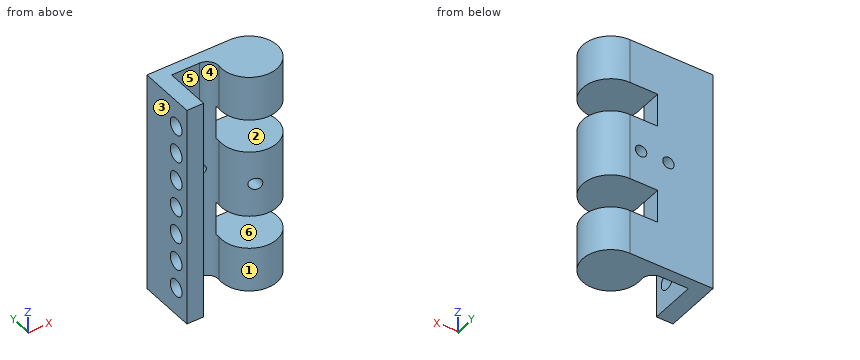
Autodesk Inventor part; units mm, degrees
ref_plane "YZ Plane" through (0, 0, 0) normal (1, 0, 0) x (0, 1, 0)
ref_plane "XZ Plane" through (0, 0, 0) normal (0, 1, 0) x (-1, 0, 0)
ref_plane "XY Plane" through (0, 0, 0) normal (0, 0, 1) x (1, 0, 0)
sketch "Sketch1" plane through (0, 0, 0) normal (1, 0, 0) x (0, 1, 0)
  line L0 (0, 0) -> (16.51, 0)
  line L1 (16.51, 0) -> (16.51, -63.5)
  line L2 (16.51, -63.5) -> (0, -63.5)
  line L3 (0, -63.5) -> (0, 0)
  circle A0 centre (4.445, -7.62) radius 2.4329
  circle A1 centre (4.445, -15.6185) radius 2.4329
  circle A2 centre (4.445, -23.6169) radius 2.4329
  circle A3 centre (4.445, -31.6154) radius 2.4329
  circle A4 centre (4.445, -39.6138) radius 2.4329
  circle A5 centre (4.445, -47.6123) radius 2.4329
  circle A6 centre (4.445, -55.6108) radius 2.4329
  dimension "d0" = 63.5
  dimension "d1" = 16.51
  dimension "d6" = 7.9985
  dimension "d11" = 7.62
extrude "Extrusion1" add sketch "Sketch1" along normal blind 4.7625
sketch "Sketch2" plane through (4.7625, 0, 0) normal (1, 0, 0) x (0, 0, -1)
  line L0 (63.5, 16.51) -> (0, 16.51)
  line L1 (63.5, 0) -> (63.5, 16.51)
  line L2 (0, 16.51) -> (63.5, 16.51)
  line L3 (63.5, 16.51) -> (63.5, 13.208)
  line L4 (63.5, 13.208) -> (0, 13.208)
  line L5 (0, 13.208) -> (0, 16.51)
  point P0 (0, 0)
  dimension "d14" = 3.302
extrude "Extrusion2" add sketch "Sketch2" along normal blind 1.016
sketch "Sketch3" plane through (0, 0, 0) normal (0, 0, 1) x (1, 0, 0)
  line L0 (5.7785, 16.51) -> (5.7785, 13.208)
  arc A0 (15.8804, 9.6157) -> (23.749, 16.51) centre (23.749, 8.5725) ccw
  line L1 (0, 16.51) -> (0, 0)
  line L2 (5.7785, 16.51) -> (23.749, 16.51)
  line L3 (4.7625, 13.208) -> (5.7785, 13.208)
  line L4 (5.7785, 13.208) -> (12.7329, 13.208)
  arc A1 (15.8804, 9.6157) -> (12.7329, 13.208) centre (12.7329, 10.033) ccw
  point P0 (17.3057, 13.208)
  point P1 (9.5258, 13.208)
  dimension "d17" = 23.749
  dimension "d18" = 15.875
  dimension "d19" = 3.175
extrude "Extrusion3" add sketch "Sketch3" against normal blind 63.5
sketch "Sketch4" plane through (0, 16.51, 0) normal (0, 1, 0) x (1, 0, 0)
  line L0 (31.6865, 0) -> (31.6865, 63.5)
  line L1 (31.6865, 0) -> (31.6865, 83.2403)
  point P0 (0, 0)
ref_plane "Work Plane1" through (55.5625, 0, 0) normal (1, 0, 0) x (0, 0, -1)
sketch "Sketch6" plane through (0, 16.51, 0) normal (0, 1, 0) x (1, 0, 0)
  line L0 (31.6865, 0) -> (31.6865, 63.5)
  line L1 (15.8115, 50.8) -> (31.6865, 50.8)
  line L2 (31.6865, 50.8) -> (31.6865, 41.275)
  line L3 (31.6865, 41.275) -> (15.8115, 41.275)
  line L4 (15.8115, 41.275) -> (15.8115, 50.8)
  line L5 (31.6865, 63.5) -> (15.8115, 63.5)
  line L6 (15.8115, 22.225) -> (31.6865, 22.225)
  line L7 (31.6865, 22.225) -> (31.6865, 12.7)
  line L8 (31.6865, 12.7) -> (15.8115, 12.7)
  line L9 (15.8115, 12.7) -> (15.8115, 22.225)
  line L10 (15.8115, 0) -> (31.6865, 0)
  point P0 (0, 0)
  point P1 (15.8804, 63.5)
  point P2 (15.8804, 0)
  dimension "d26" = 9.525
  dimension "d27" = 12.7
  dimension "d28" = 9.525
  dimension "d29" = 12.7
  dimension "d32" = 15.875
  dimension "d33" = 15.875
extrude "Extrusion4" cut sketch "Sketch6" against normal through all
sketch "Sketch7" plane through (0, 16.51, 0) normal (0, 1, 0) x (1, 0, 0)
  circle A0 centre (20.574, 31.75) radius 1.6383
  line L0 (0, 0) -> (23.749, 0)
  line L1 (23.749, 22.225) -> (23.749, 41.275)
  line L2 (12.7329, 0) -> (12.7329, 63.5)
  circle A1 centre (12.7329, 31.75) radius 1.6383
  dimension "d34" = 3.2766
  dimension "d35" = 31.75
  dimension "d36" = 3.175
  dimension "d37" = 3.2766
extrude "Extrusion5" cut sketch "Sketch7" against normal through all
properties part number "knuckle plate hinge tall"
Here's how the part is built. I have some questions about the finished solid (model axes, mm). Face numbers are marked on the shaded views. A direction names the side the tool comes from. Give positions to 0.01 mm unless a question says otherwise; leave off trailing zeros. Order: outer loops, then holes, each group sorted by start corner. A loop starts at its lowest first (then second) coordinate and runs counter-clockwise, first axis right, second up. Notation, with made-up numbers: (85.5, -33) -> (108.5, -33) arc R15 ccw to (108.5, -14) -> close; hole circle Ø7 at (64.5, -36). An arc over 180 degrees is marked (long way). Use CSV: the item, a comma, the result in double quotes. Start each with the question number.
Item 1: Suppose I cut it at C-C (z = -36.5). List the corners of the cut face in (x, y) for me.
Item 2: Suppose I cut it at D-D (x = 4). List the corners of the cut face in (y, z) for me (1 decimal).
Item 3: Suppose I cut it at A-A (z = -7.62). List the corners of the cut face in (x, y) for me.
Item 4: Thinking about a two-plate mould opening in X: for the marked faces 1, 2 and 3, which applies, pulls with the +X half, pulls with the -X half, needs draft (parallel to the pull), parting line crosses it, or undercut?
Item 5: On a 3-axis mill with a long thin cutter (end or side, diameter ignored), from which of +Z, -Z, +X, -X, +Y, -Y can I reach the whole of each face in a straight line? I mean the marked faces 4, 5 and 6. Say none if no direction works.
Item 6: Suppose I cut it at B-B (x = 17). List the corners of the cut face in (y, z) for me (3 decimals), and give its area (3 significant figures).
Item 7: If I drill on probe 1 along Z at (x, y) = (28, 7.5) (3 decimals); probe 2 along X at (y, z) = (8.75, -31.75); probe 3 along Z at (x, y) = (20, 6) (3 decimals), over which ranges is the centre line in solid material (lowest first)? Write a range as [from, to].
Item 8: I'm going to push flat-ended pins straight in: P1, Ø6.5, axis at y = 14, z = -46.5, coming from the +X side; P2, Ø2, axis at x = 20.574, z = -31.75, coming from the -Y side; P3, Ø8, axis at y = 4.44, z = -31.62, coming from the -X side; P4, Ø2, axis at x = 20.5, z = -36.5, coming from the -Y side. Where does each tip first touch, or does it pass through?
Answer block:
1,outline,"(0, 0) -> (4.76, 0) -> (4.76, 13.21) -> (12.73, 13.21) arc R3.17 cw to (15.88, 9.62) arc R7.94 ccw (long way) to (23.75, 16.51) -> (0, 16.51) -> close"
2,outline,"(0, -63.5) -> (16.5, -63.5) -> (16.5, 0) -> (0, 0) -> close; hole circle Ø4.9 at (4.4, -55.6); hole circle Ø4.9 at (4.4, -47.6); hole circle Ø4.9 at (4.4, -39.6); hole circle Ø4.9 at (4.4, -31.6); hole circle Ø4.9 at (4.4, -23.6); hole circle Ø4.9 at (4.4, -15.6); hole circle Ø4.9 at (4.4, -7.6)"
3,outline,"(0, 0) -> (4.76, 0) -> (4.76, 2.01) -> (0, 2.01) -> close; (0, 6.88) -> (4.76, 6.88) -> (4.76, 13.21) -> (12.73, 13.21) arc R3.17 cw to (15.88, 9.62) arc R7.94 ccw (long way) to (23.75, 16.51) -> (0, 16.51) -> close"
4,face 1,"undercut"
4,face 2,"needs draft"
4,face 3,"pulls with the -X half"
5,face 4,"+Z, -Z"
5,face 5,"+Z, -Z, -Y"
5,face 6,"+X, +Y, -Y"
6,outline,"(4.395, -63.5) -> (16.51, -63.5) -> (16.51, -50.8) -> (4.395, -50.8) -> close; (4.395, -41.275) -> (16.51, -41.275) -> (16.51, -22.225) -> (4.395, -22.225) -> close; (4.395, -12.7) -> (16.51, -12.7) -> (16.51, 0) -> (4.395, 0) -> close"
6,area,"539 mm^2"
7,probe 1,"z = [-63.5, -50.8], [-41.275, -22.225], [-12.7, 0]"
7,probe 2,"x = [0, 4.76], [15.81, 18.94], [22.21, 31.68]"
7,probe 3,"z = [-63.5, -50.8], [-41.275, -33.284], [-30.216, -22.225], [-12.7, 0]"
8,P1,"stops at x = 15.81"
8,P2,"passes through"
8,P3,"stops at x = 0"
8,P4,"stops at y = 0.96"
